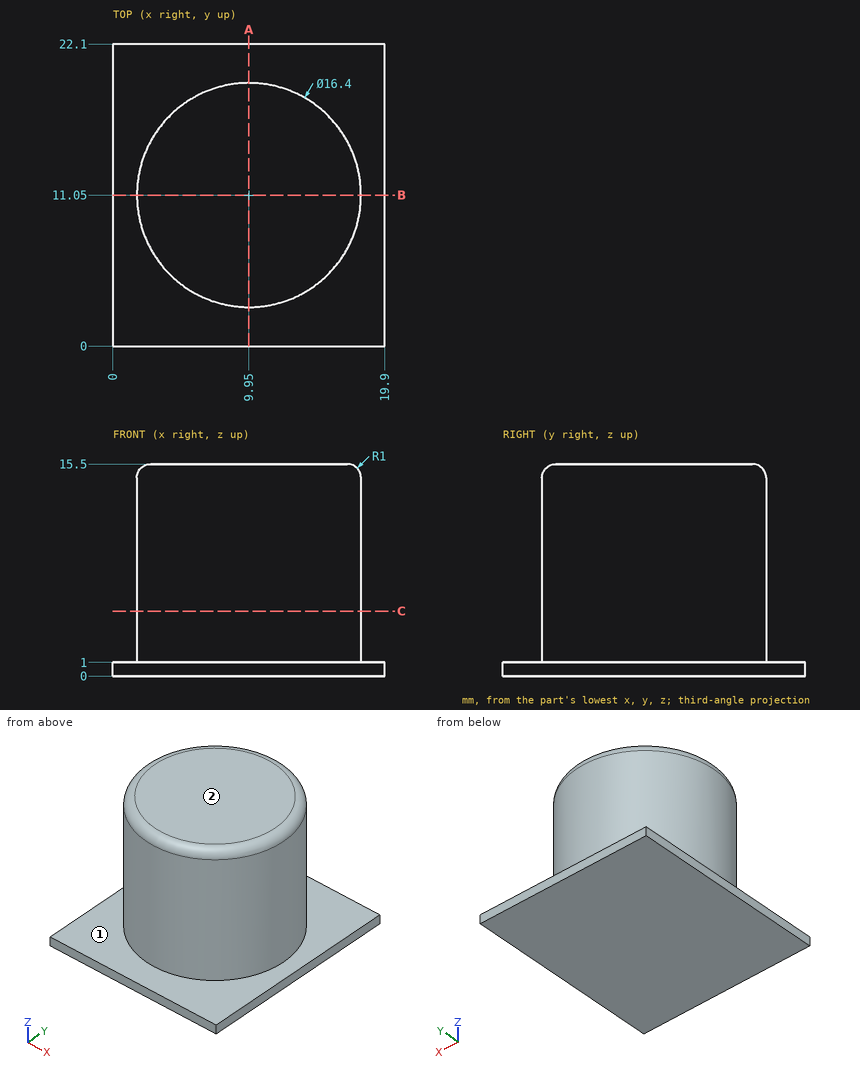
Answer from the drawing. Dimensions are ordinates in mm from the lowest x, y and z of the part. A direction names the side the tool comes from. Coordinates: 2 decimals unless noted, no trailing zeros. Loops run counter-clockwise (first coordinate to the right, second up) from the corner with the lowest first, then second, coordinate; pieces in that order, holes last.
1) Section B-B (y = 11.05) is taken. Give the vertices of the cut face in (x, z).
Results:
outline: (0, 0) - (19.9, 0) - (19.9, 1) - (18.15, 1) - (18.15, 14.5) arc R1 ccw to (17.15, 15.5) - (2.75, 15.5) arc R1 ccw to (1.75, 14.5) - (1.75, 1) - (0, 1) - close
2) For the marked faces 1 and 2, determine the directions among +Z, -Z, +X, -X, +Y, -Y from which every point of the face is accessible in a straight line to the end or side of a thin tool.
Results:
face 1: +Z
face 2: +Z, +X, -X, +Y, -Y
3) Section C-C (z = 4.75) is taken. Give the vertices of the cut face in (x, y), plus the area to 3 significant figures.
Results:
outline: circle Ø16.4 at (9.95, 11.05)
area: 211 mm2
4) Consider probe 1 along Z at (x, y) = (4.25, 19.75); probe 2 along Y at (x, z) = (4, 2.25); probe 3 along X at (y, z) = (7.5, 14.5). Determine where each line is inside the solid, lowest interval first.
Results:
probe 1: z = 0 to 1
probe 2: y = 5.41 to 16.69
probe 3: x = 2.56 to 17.34
5) Section A-A (x = 9.95) is taken. Give the vertices of the cut face in (y, z), plus the area to 3 significant figures.
Results:
outline: (0, 0) - (22.1, 0) - (22.1, 1) - (19.25, 1) - (19.25, 14.5) arc R1 ccw to (18.25, 15.5) - (3.85, 15.5) arc R1 ccw to (2.85, 14.5) - (2.85, 1) - (0, 1) - close
area: 259 mm2
6) Flat-ended cylindrical pins translate along their axes: pin 1 (3 mm diameter, centred on x = 16, z = 14, fed in from +Y); pin 2 (4 mm diameter, centred on x = 10, z = 12, fed in from +Y); pin 3 (5 mm diameter, centred on y = 10.5, z = 8, fed in from +X). Find the tip coordinate at first contact, or state that the pin passes through.
Results:
pin 1: stops at y = 17.87
pin 2: stops at y = 19.25
pin 3: stops at x = 18.15
